Drawing for the job (mm, zero at the part's lowest x, y, z). Give positions to 0.01 mm unless a question says otherwise; leave off trailing zeros. Loops run counter-clockwise (first coordinate to the right, second up) from the corner with the lowest first, then second, coordinate; pieces in that order, holes last. Notation, with made-up numbers: (62, 88) -> (90, 88) arc R12 ccw to (90, 100) -> close; hole circle Ø7 at (40, 68). An arc over 180 degrees is marked (long way). Use CSV: the item, a comma, the result in double quotes. Start each with the question number.
(1) Cut at C-C on x = 40.5. Write the cut outline in (y, z).
(2) Cut at A-A on y = 7. Write the cut outline in (x, z).
(3) Cut at B-B on z = 2. Write the cut outline in (x, y) (3 decimals).
(4) Drill centre lines: probe 1 along Y at (x, z) = (39, 0.6); probe 2 along X at (y, z) = (8.75, 2.1); probe 3 along X at (y, z) = (5.5, 1.1). Where is each one in solid material? Low to high.
(5) Cut at D-D on y = 11. Write the cut outline in (x, z) (3 decimals).
(6) Flat gauge pins, fed straight in: pin 1 (1 mm diameter, centred on x = 37.5, z = 0.5, fed in from +Y); pin 2 (1.5 mm diameter, centred on y = 6.5, z = 1.5, fed in from -X); pin 3 (0.9 mm diameter, centred on y = 5, z = 1.5, fed in from +X). Where does each tip first touch, or does it go through?
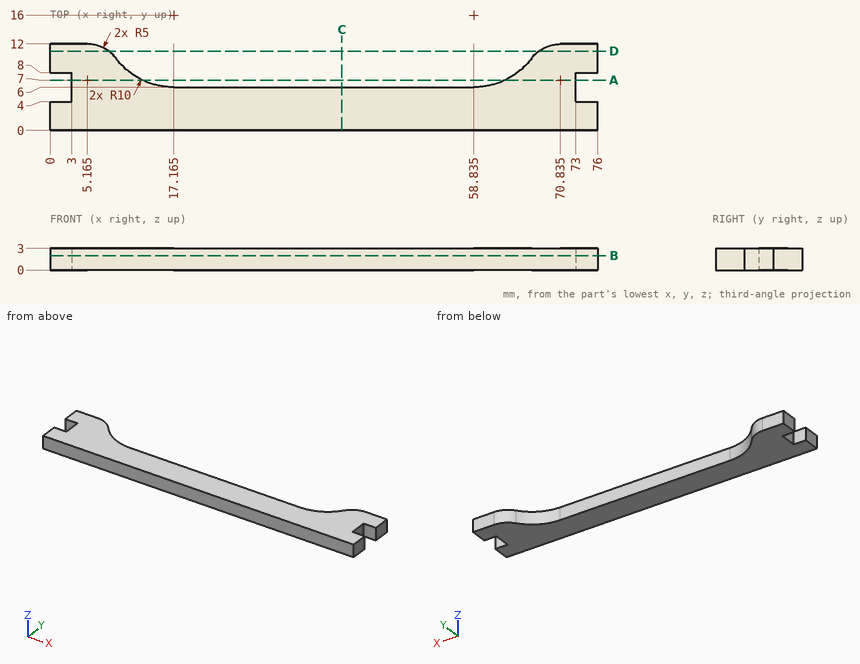
Check result:
1,outline,"(0, 0) -> (6, 0) -> (6, 3) -> (0, 3) -> close"
2,outline,"(3, 0) -> (12.81, 0) -> (12.81, 3) -> (3, 3) -> close; (63.19, 0) -> (73, 0) -> (73, 3) -> (63.19, 3) -> close"
3,outline,"(0, 0) -> (76, 0) -> (76, 4) -> (73, 4) -> (73, 8) -> (76, 8) -> (76, 12) -> (70.835, 12) arc R5 ccw to (66.835, 10) arc R10 cw to (58.835, 6) -> (17.165, 6) arc R10 cw to (9.165, 10) arc R5 ccw to (5.165, 12) -> (0, 12) -> (0, 8) -> (3, 8) -> (3, 4) -> (0, 4) -> close"
4,probe 1,"0 to 6"
4,probe 2,"0 to 10.28, 65.72 to 76"
4,probe 3,"3 to 73"
5,outline,"(0, 0) -> (8.165, 0) -> (8.165, 3) -> (0, 3) -> close; (67.835, 0) -> (76, 0) -> (76, 3) -> (67.835, 3) -> close"
6,pin 1,"y = 6"
6,pin 2,"x = 3"
6,pin 3,"x = 73"
